```python
from build123d import *

# Parameters (mm, degrees)
F1_DEPTH = 5
F3_DEPTH = 180
F5_DEPTH = 5
F7_D     = 3
F7_DEPTH = 200
F7_TIP   = 0.9012909285


with BuildPart() as f1:
    # F0 (on Top) → F1 (new body)
    with BuildSketch(Plane.XY):
        with BuildLine():
            Line((-75, 0), (0, 0))
            Line((0, 0), (75, 0))
            ThreePointArc((75, 0), (3.0622988388, 32.2584255386), (-75, 43.3))
            Line((-75, 43.3), (-75, 0))
        make_face()
    extrude(amount=F1_DEPTH)

    # F2 (on face) → F3 (join)
    with BuildSketch(Plane.XY.offset(5)):
        with BuildLine():
            ThreePointArc((75, 0), (3.0622988388, 32.2584255386), (-75, 43.3))
            Line((-75, 43.3), (-75, 38.3))
            ThreePointArc((-75, 38.3), (-0.0135178849, 28.5635745872), (70, 0))
            Line((70, 0), (75, 0))
        make_face()
    extrude(amount=F3_DEPTH)

    # F4 (on face) → F5 (join)
    with BuildSketch(Plane.XY.offset(185)):
        with BuildLine():
            ThreePointArc((70, 0), (-0.0135178849, 28.5635745872), (-75, 38.3))
            Line((-75, 38.3), (-75, 0))
            Line((-75, 0), (70, 0))
        make_face()
        with BuildLine():
            Line((-75, 43.3), (-75, 38.3))
            ThreePointArc((-75, 38.3), (-0.0135178849, 28.5635745872), (70, 0))
            Line((70, 0), (75, 0))
            ThreePointArc((75, 0), (3.0622988388, 32.2584255386), (-75, 43.3))
        make_face()
    extrude(amount=F5_DEPTH)

    # F7
    with Locations(Plane.XY.offset(190)):
        with Locations((-65, 30), (-65, 10)):
            Hole(F7_D / 2, depth=F7_DEPTH)
            with Locations((0, 0, -(F7_DEPTH + F7_TIP / 2))):  # 118° drill point
                Cone(0, F7_D / 2, F7_TIP, mode=Mode.SUBTRACT)


solid = f1.part
```
Check sheet for the modelled part. Datum: model origin and axes. Units: mm. A direction names the side the tool comes from. Give positions to 0.01 mm unless a question says otherwise; leave off trailing zeros. Loops run counter-clockwise (first coordinate to the right, second up) from the corner with the lowest first, then second, coordinate; pieces in that order, holes last. Notation, with made-up numbers: (42.5, 69) - (79.5, 69) arc R21 cw to (79.5, 87) - close; hole circle Ø11 at (-23.5, 11). An arc over 180 degrees is marked (long way). One line per question, with ' | ' between items. Start each with the question number.
1. Gauge pin test, flat ends, axial feed: pin 1 Ø12 at (x, z) = (-35.5, 133) entering from -Y; pin 2 Ø6 at (x, z) = (40, 112) entering from -Y; pin 3 Ø10 at (x, z) = (-2.5, 120) entering from -Y. Record the tip position at first contact, or that the pin passes through.
2. Set-up check for faces 1 (the cylindrical face through (4.13, 31.95, 93.67)), 2 (the cylindrical face through (-1.04, 28.833, 93.74)): record each of +Z, -Z, +X, -X, +Y, -Y from which the full face is reachable in a straight line by a thin tool's end or side.
3. Draft check along Z on faces 3 (the flat face through (-75, 39, 95)), 4 (the flat face through (-18, 17, 0)), 5 (the flat face through (-20, 15, 185)). Enter one of: released by +Z, released by -Z, zero draft, split by the parting line, or undercut.
4. Material ranges on line 1 along Z through (x, y) = (4, 19); line 2 along Y through (x, z) = (-65, 1); line 3 along X through (y, z) = (14, 105.5), recorded low to high. Write a range as [from, to].
5. Cross-section at B-B, the plane x = -14. Enter the section's corners in (y, z).
6. Cross-section at A-A, the plane y = 20.5. Enter the section's corners in (x, z), plus the area to 3 significant figures.
7. Cross-section at C-C, the plane z = 11. Enter the section's corners in (x, y).
Check result:
1) pin 1: stops at y = 34.75 | pin 2: stops at y = 13.55 | pin 3: stops at y = 27.89
2) face 1: +Z, -Z, +X, +Y | face 2: -X, -Y
3) face 3: zero draft | face 4: released by -Z | face 5: undercut
4) line 1: z = [0, 5], [185, 190] | line 2: y = [0, 8.5], [11.5, 28.5], [31.5, 43.12] | line 3: x = [41.96, 50.04]
5) outline: (0, 0) - (36.61, 0) - (36.61, 190) - (0, 190) - (0, 185) - (31.89, 185) - (31.89, 5) - (0, 5) - close
6) outline: (-75, 0) - (35.97, 0) - (35.97, 190) - (-75, 190) - (-75, 185) - (25.68, 185) - (25.68, 5) - (-75, 5) - close | area: 2,960 mm2
7) outline: (-75, 38.3) arc R293.63 cw to (70, 0) - (75, 0) arc R281.47 ccw to (-75, 43.3) - close
